```python
from build123d import *

# Parameters (mm, degrees)
MOUNT_DEPTH            = 10
IZIM5_W                = 14.5
IZIM5_H                = 2
MOTOR_ST_DEPTH         = 6
C_VATA_START           = -2
IZIM6_R                = 1.6
C_VATA_DELIKLERI_DEPTH = 6
IZIM7_R                = 2.85
KES_EKSTR_ZYON1_DEPTH  = 8.9


with BuildPart() as part:
    # Çizim4 → mount (new body)
    with BuildSketch(Plane.XY):
        Polygon((-22, 2.1), (-14, 2.1), (-14, 12), (15, 12), (15, 3.1), (23, 3.1), (23, 1.1), (13, 1.1), (13, 10), (-12, 10), (-12, 0.1), (-22, 0.1), align=None)
    extrude(amount=MOUNT_DEPTH)

    # Çizim5 → motor üstü (add)
    with BuildSketch(Plane.XY.offset(10)):
        with Locations((-6.75, 11)):
            Rectangle(IZIM5_W, IZIM5_H)
    extrude(amount=MOTOR_ST_DEPTH)

    # Çizim6 → cıvata delikleri (cut)
    with BuildSketch(Plane(origin=(0, 2.1, 0), x_dir=(1, 0, 0), z_dir=(0, 1, 0)).offset(C_VATA_START)):
        with Locations(Location((-18, -5, 0), (0, 0, 270))):
            Circle(IZIM6_R)
        with Locations(Location((16.7, -5, 0), (0, 0, 180))):
            Circle(IZIM6_R)
    extrude(amount=C_VATA_DELIKLERI_DEPTH, mode=Mode.SUBTRACT)

    # Çizim7 → Kes-Ekstrüzyon1 (cut)
    with BuildSketch(Plane(origin=(0, 3.1, 0), x_dir=(1, 0, 0), z_dir=(0, 1, 0))):
        with Locations((16.7, -5)):
            Circle(IZIM7_R)
    extrude(amount=KES_EKSTR_ZYON1_DEPTH, mode=Mode.SUBTRACT)


solid = part.part
```
Geometry check sheet. Reference: the model listing, model coordinates, mm. A direction names the side the tool comes from. Coordinates: 2 decimals unless noted, no trailing zeros. Order: outer loops, then holes, each group sorted by start corner. A loop starts at its lowest first (then second) coordinate and runs counter-clockwise, first axis right, second up.
Item 1: Section check D-D (z = 1.75). Enter the section's corners in (x, y).
Item 2: Depth check by flat-ended pin: pin 1 (5.5 mm diameter, centred on x = 10.5, y = 6.5, fed in from +Z); pin 2 (3 mm diameter, centred on y = 8.5, z = 7.5, fed in from -X); pin 3 (3 mm diameter, centred on y = 7, z = 8.5, fed in from +X). Enter the tip coordinate at first touch or a pass-through.
Item 3: Section check C-C (z = 5). Enter the section's corners in (x, y).
Item 4: Section check B-B (x = -18). Enter the section's corners in (y, z).
Item 5: Scan lines: line 1 along Z through (x, y) = (-18, 1.4); line 2 along Y through (x, z) = (-18.5, 7.75); line 3 along Y through (x, z) = (6, 7.5). Record each from-to range of solid material in increasing order.
Item 6: Section check A-A (y = 6). Enter the section's corners in (x, z), plus the area to 3 significant figures.
Item 7: Mould release check, pull along Z, two halves, no side actions. Record for faces 6 (the flat face through (-14.7, 1.8, 10)), 7 (the cylindrical face through (-16.414, 1.086, 4.792)), 8 (the flat face through (-22, 1, 5)): released by +Z, released by -Z, zero draft, split by the parting line, or undercut.
Item 8: Tool access check on faces 1 (the flat face through (19, 1.1, 5)), 2 (the flat face through (0.5, 11, 13)), 3 (the flat face through (-12, 5, 5)), 4 (the flat face through (-16, 2.1, 5)), 5 (the flat face through (15, 8, 9)). Record the directions out of +Z, -Z, +X, -X, +Y, -Y that give a thin tool (end or side, any length) a straight path to the whole face; none if there is none.
Check sheet entries:
1. outline: (-22, 0.1) - (-12, 0.1) - (-12, 10) - (13, 10) - (13, 1.1) - (23, 1.1) - (23, 3.1) - (15, 3.1) - (15, 12) - (-14, 12) - (-14, 2.1) - (-22, 2.1) - close
2. pin 1: stops at z = 10
2. pin 2: stops at x = -14
2. pin 3: stops at x = 15
3. outline: (-22, 0.1) - (-19.6, 0.1) - (-19.6, 2.1) - (-22, 2.1) - close; (-16.4, 0.1) - (-12, 0.1) - (-12, 10) - (13, 10) - (13, 1.1) - (15.1, 1.1) - (15.1, 3.1) - (13.85, 3.1) - (13.85, 12) - (-14, 12) - (-14, 2.1) - (-16.4, 2.1) - close; (18.3, 1.1) - (23, 1.1) - (23, 3.1) - (18.3, 3.1) - close
4. outline: (0.1, 0) - (2.1, 0) - (2.1, 3.4) - (0.1, 3.4) - close; (0.1, 6.6) - (2.1, 6.6) - (2.1, 10) - (0.1, 10) - close
5. line 1: z = 0 to 3.4, 6.6 to 10
5. line 2: y = 0.1 to 2.1
5. line 3: y = 10 to 12
6. outline: (-14, 0) - (-12, 0) - (-12, 10) - (-14, 10) - close; (13, 0) - (15, 0) - (15, 2.71) arc R2.85 cw to (15, 7.29) - (15, 10) - (13, 10) - close
6. area: 36.3 mm2
7. face 6: released by +Z
7. face 7: undercut
7. face 8: zero draft
8. face 1: +Z, -Z, +X, -Y
8. face 2: +Z, +X, +Y, -Y
8. face 3: +Z, -Z, -Y
8. face 4: +Z, -Z, -X, +Y
8. face 5: +Z, -Z, +X, +Y
